Check sheet for the drawn part. Datum: minimum x, y, z corner. Units: mm. A direction names the side the tool comes from. Give positions to 0.01 mm unless a question says otherwise; leave off trailing zeros. Order: outer loops, then holes, each group sorted by start corner. A loop starts at its lowest first (then second) coordinate and runs counter-clockwise, first axis right, second up. Notation, with made-up numbers: M 77,1.5 L 91,1.5 A22 ccw 91,39.5 Z; hole C 86.25,71 d3. An arc over 180 degrees is marked long. One line per question, with ' | ' between items. Start each with the question number.
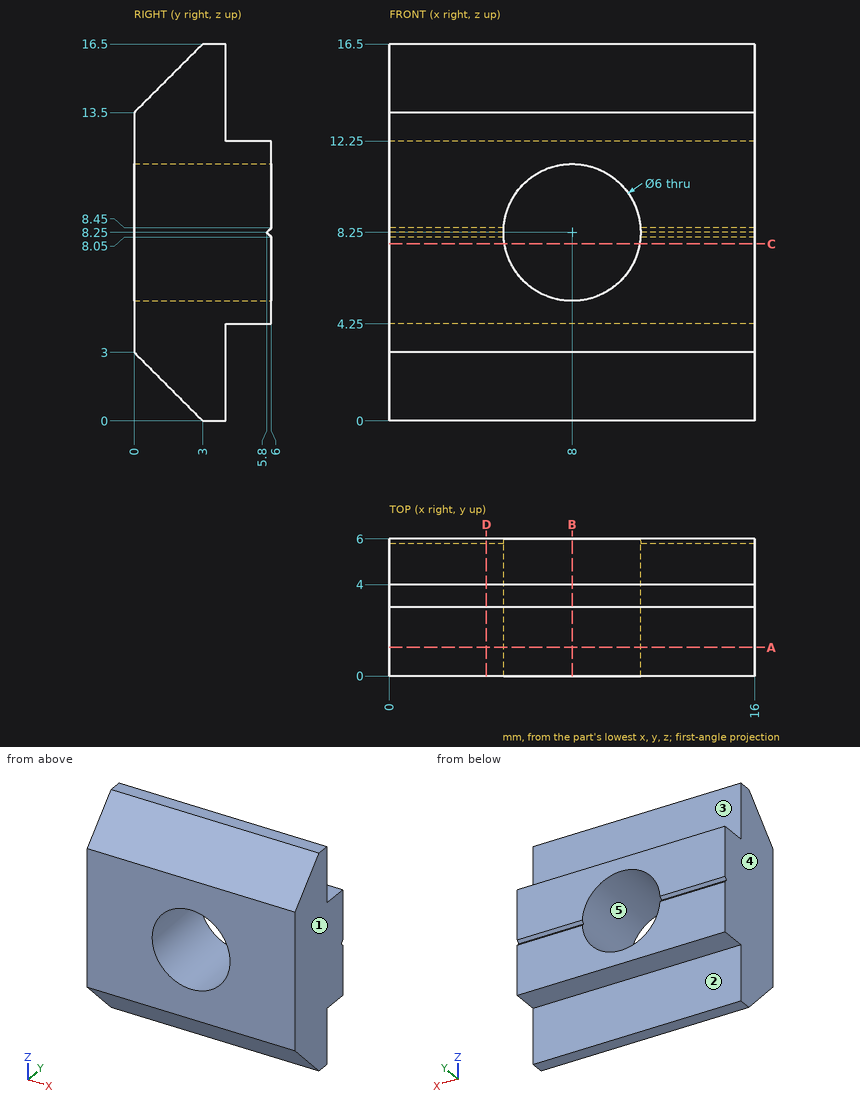
Item 1: Section check D-D, the plane x = 4.25. Record the cut outline in (y, z).
Item 2: Set-up check for the marked faces 1 and 2: record each of +Z, -Z, +X, -X, +Y, -Y from which the full face is reachable in a straight line by a thin tool's end or side.
Item 3: Go/stop test with flat-tipped pins: P1, Ø2, axis at x = 7, z = 14.5, coming from the +Y side; P2, Ø6, axis at x = 8, z = 13.5, coming from the -Y side; P3, Ø1.5, axis at x = 7, z = 2, coming from the -Y side; P4, Ø2, axis at x = 5.5, y = 0.5, coming from the +Z side. Record where each tip stops, or that it passes through.
Item 4: Scan lines: probe 1 along Z at (x, y) = (8, 3.5); probe 2 along X at (y, z) = (4, 8.25); probe 3 along Z at (x, y) = (8, 4.75). Record each from-to range of solid material in increasing order. Write a range as [from, to].
Item 5: Draft check along X on the marked faces 3, 4 and 5. Enter one of: released by +X, released by -X, zero draft, split by the parting line, or undercut.
Item 6: Section check A-A, the plane y = 1.25. Record the cut outline in (x, z), then the cut area to 3 significant figures.
Item 7: Section check C-C, the plane z = 7.75. Record the cut outline in (x, y).
Item 8: Section check B-B, the plane x = 8. Record the cut outline in (y, z), then the cut area to 3 significant figures.
Reported:
1) outline: M 0,3 L 3,0 L 4,0 L 4,4.25 L 6,4.25 L 6,8.05 L 5.8,8.25 L 6,8.45 L 6,12.25 L 4,12.25 L 4,16.5 L 3,16.5 L 0,13.5 Z
2) face 1: +Z, -Z, +X, +Y, -Y | face 2: -Z, +X, -X, +Y
3) P1: stops at y = 4 | P2: stops at y = 0 | P3: stops at y = 0.25 | P4: stops at z = 15
4) probe 1: z = [0, 5.25], [11.25, 16.5] | probe 2: x = [0, 5], [11, 16] | probe 3: z = [4.25, 5.25], [11.25, 12.25]
5) face 3: zero draft | face 4: released by -X | face 5: undercut
6) outline: M 0,1.75 L 16,1.75 L 16,14.75 L 0,14.75 Z; hole C 8,8.25 d6 | area: 180 mm^2
7) outline: M 0,0 L 5.04,0 L 5.04,6 L 0,6 Z; M 10.96,0 L 16,0 L 16,6 L 10.96,6 Z
8) outline: M 0,3 L 3,0 L 4,0 L 4,4.25 L 6,4.25 L 6,5.25 L 0,5.25 Z; M 0,11.25 L 6,11.25 L 6,12.25 L 4,12.25 L 4,16.5 L 3,16.5 L 0,13.5 Z | area: 37.0 mm^2
